from build123d import *

# Parameters (mm, degrees)
ESBO_O1_W                = 40
ESBO_O1_H                = 40
RESSALTO_EXTRUS_O1_DEPTH = 10
RESSALTO_EXTRUS_O2_DEPTH = 136
ESBO_O3_W                = 30
ESBO_O3_H                = 10
RESSALTO_EXTRUS_O3_DEPTH = 30
ESBO_O4_W                = 30
ESBO_O4_H                = 4
CORTE_EXTRUS_O1_DEPTH    = 11


with BuildPart() as part:
    # Esboço1 → Ressalto-extrusão1 (new body)
    with BuildSketch(Plane(origin=(0, 0, 0), x_dir=(1, 0, 0), z_dir=(0, 1, 0))):
        with Locations((20, -20)):
            Rectangle(ESBO_O1_W, ESBO_O1_H)
    extrude(amount=RESSALTO_EXTRUS_O1_DEPTH)

    # Esboço2 → Ressalto-extrusão2 (add)
    with BuildSketch(Plane(origin=(0, 10, 0), x_dir=(1, 0, 0), z_dir=(0, 1, 0))):
        Polygon((40, 0), (30, 0), (30, -30), (0, -30), (0, -40), (40, -40), align=None)
    extrude(amount=RESSALTO_EXTRUS_O2_DEPTH)

    # Esboço3 → Ressalto-extrusão3 (add)
    with BuildSketch(Plane(origin=(0, 0, 30), x_dir=(-1, 0, 0), z_dir=(0, 0, -1))):
        with Locations((-15, 141)):
            Rectangle(ESBO_O3_W, ESBO_O3_H)
        with Locations((-15, 127)):
            Rectangle(ESBO_O3_W, ESBO_O3_H)
    extrude(amount=RESSALTO_EXTRUS_O3_DEPTH)

    # Esboço4 → Corte-extrusão1 (cut, through all)
    with BuildSketch(Plane(origin=(0, 0, 30), x_dir=(-1, 0, 0), z_dir=(0, 0, -1))):
        with Locations((-15, 134)):
            Rectangle(ESBO_O4_W, ESBO_O4_H)
    extrude(amount=-CORTE_EXTRUS_O1_DEPTH, mode=Mode.SUBTRACT)


solid = part.part
Geometry: final body of the model. Coordinates: model frame, mm. A direction names the side the tool comes from. Give positions to 0.01 mm unless a question says otherwise; leave off trailing zeros. Order: outer loops, then holes, each group sorted by start corner. A loop starts at its lowest first (then second) coordinate and runs counter-clockwise, first axis right, second up. Notation, with made-up numbers: (76.25, -20.5) -> (134.25, -20.5) arc R14 ccw to (134.25, 3.5) -> close; hole circle Ø7 at (6.25, 85.5). An arc over 180 degrees is marked (long way). Put each result on its own line as item: value.
Q1. Section A-A, the plane x = 18. Return loops of the section in (y, z).
Here are the results:
outline: (0, 0) -> (10, 0) -> (10, 30) -> (122, 30) -> (122, 0) -> (132, 0) -> (132, 40) -> (0, 40) -> close; (136, 0) -> (146, 0) -> (146, 40) -> (136, 40) -> close
Q2. Section D-D, the plane z = 19.5. Return loops of the section in (x, y), then the cut area to 3 significant figures.
Here are the results:
outline: (0, 0) -> (40, 0) -> (40, 146) -> (0, 146) -> (0, 136) -> (30, 136) -> (30, 132) -> (0, 132) -> (0, 122) -> (30, 122) -> (30, 10) -> (0, 10) -> close
area: 2,360 mm^2
Q3. Section B-B, the plane z = 32.5. Return loops of the section in (x, y).
Here are the results:
outline: (0, 0) -> (40, 0) -> (40, 146) -> (0, 146) -> (0, 136) -> (30, 136) -> (30, 132) -> (0, 132) -> close
Q4. Draft query along Y for faces 1 (the face through (20, 146, 20)), 2 (the face through (15, 122, 15)), 3 (the face through (0, 141, 20)), 4 (the face through (15, 65, 30)). Return one class per face: released by +Y, released by -Y, zero draft, split by the parting line, or undercut.
Here are the results:
face 1: released by +Y
face 2: undercut
face 3: zero draft
face 4: undercut
Q5. Reachability of faces 5 (the face through (20, 0, 20)), 6 (the face through (15, 10, 15)), 7 (the face through (15, 136, 20)) from +Z, -Z, +X, -X, +Y, -Y: full face, straight path, thin tool, end or side. Return the list, or none.
Here are the results:
face 5: +Z, -Z, +X, -X, -Y
face 6: -Z, -X
face 7: +Z, -Z, -X
Q6. Pin query (flat end, axial travel): pin 1 (3 mm diameter, centred on y = 70.5, z = 17.5, fed in from -X); pin 2 (24 mm diameter, centred on x = 12, y = 88.5, fed in from -Z). Return the tip coordinate at first contact, or that it passes through.
Here are the results:
pin 1: stops at x = 30
pin 2: stops at z = 30
Q7. Material intervals for L1, parallel to Y at x = 14.5, z = 18.5; L2, parallel to Y at x = 23.5, z = 37.5; L3, parallel to Z at x = 7, y = 23.5, sorted ascending.
Here are the results:
L1: y = 0 to 10, 122 to 132, 136 to 146
L2: y = 0 to 132, 136 to 146
L3: z = 30 to 40
Q8. Section C-C, the plane y = 51.5. Return loops of the section in (x, z), then the cut area to 3 significant figures.
Here are the results:
outline: (0, 30) -> (30, 30) -> (30, 0) -> (40, 0) -> (40, 40) -> (0, 40) -> close
area: 700 mm^2
